Can you work these out from the model? Positions are in its coordinate system, mm. A direction names the side the tool comes from. Coordinates: 2 decimals unless noted, no trailing zeros. Write each loop counter-clockwise with the first axis right and the second up, starting at its lowest first coordinate (ties: lowest second). Pieces come first, ordered by that corner, then holes. Notation, with made-up numbers: (-19.5, 8) -> (9.5, 8) arc R34 cw to (9.5, 40) -> close; hole circle Ø8 at (23.5, 71). An arc over 180 degrees is marked (long way). Use one line per item in the form item = value.
```python
from build123d import *

# Parameters (mm, degrees)
SKETCH1_R           = 1
SKETCH1_R_2         = 0.9
SKETCH1_R_3         = 7.5
BOSS_EXTRUDE1_DEPTH = 1.5
FILLET1_R           = 0.5
CHAMFER1_SIZE       = 0.6


with BuildPart() as part:
    # Sketch1 → Boss-Extrude1 (new body)
    with BuildSketch(Plane(origin=(0, 0, 0), x_dir=(1, 0, 0), z_dir=(0, 1, 0))):
        with BuildLine():
            Line((-10.214212529, -2.433076738), (-12.325317547, -3.651923789))
            ThreePointArc((-12.325317547, -3.651923789), (-13.423393759, -7.75), (-9.325317547, -8.848076211))
            Line((-9.325317547, -8.848076211), (-7.214212529, -7.629229161))
            ThreePointArc((-7.214212529, -7.629229161), (-5.25, -9.09326674), (-3, -10.062305899))
            Line((-3, -10.062305899), (-3, -12.5))
            ThreePointArc((-3, -12.5), (0, -15.5), (3, -12.5))
            Line((3, -12.5), (3, -10.062305899))
            ThreePointArc((3, -10.062305899), (5.25, -9.09326674), (7.214212529, -7.629229161))
            Line((7.214212529, -7.629229161), (9.325317547, -8.848076211))
            ThreePointArc((9.325317547, -8.848076211), (13.423393759, -7.75), (12.325317547, -3.651923789))
            Line((12.325317547, -3.651923789), (10.214212529, -2.433076738))
            ThreePointArc((10.214212529, -2.433076738), (10.410171044, -1.370525018), (10.495898275, -0.293461075))
            Line((10.495898275, -0.293461075), (12.850529964, 0.337460585))
            ThreePointArc((12.850529964, 0.337460585), (14.971850307, 4.011695199), (11.297615693, 6.133015543))
            Line((11.297615693, 6.133015543), (8.942984004, 5.502093883))
            ThreePointArc((8.942984004, 5.502093883), (6.391995005, 8.330210073), (3, 10.062305899))
            Line((3, 10.062305899), (3, 12.5))
            ThreePointArc((3, 12.5), (0, 15.5), (-3, 12.5))
            Line((-3, 12.5), (-3, 10.062305899))
            ThreePointArc((-3, 10.062305899), (-6.391995005, 8.330210073), (-8.942984004, 5.502093883))
            Line((-8.942984004, 5.502093883), (-11.297615693, 6.133015543))
            ThreePointArc((-11.297615693, 6.133015543), (-14.971850307, 4.011695199), (-12.850529964, 0.337460585))
            Line((-12.850529964, 0.337460585), (-10.495898275, -0.293461075))
            ThreePointArc((-10.495898275, -0.293461075), (-10.410171044, -1.370525018), (-10.214212529, -2.433076738))
        make_face()
        with Locations(Location((0, -12.5, 0), (0, 0, 270))):
            Circle(SKETCH1_R, mode=Mode.SUBTRACT)
        with Locations(Location((-10.825317547, -6.25, 0), (0, 0, 270))):
            Circle(SKETCH1_R_2, mode=Mode.SUBTRACT)
        with Locations(Location((10.825317547, -6.25, 0), (0, 0, 270))):
            Circle(SKETCH1_R_2, mode=Mode.SUBTRACT)
        with Locations(Location((0, 0, 0), (0, 0, 270))):
            Circle(SKETCH1_R_3, mode=Mode.SUBTRACT)
        with Locations(Location((0, 12.5, 0), (0, 0, 270))):
            Circle(SKETCH1_R_2, mode=Mode.SUBTRACT)
        with Locations(Location((12.074072829, 3.235238064, 0), (0, 0, 270))):
            Circle(SKETCH1_R, mode=Mode.SUBTRACT)
        with Locations(Location((-12.074072829, 3.235238064, 0), (0, 0, 270))):
            Circle(SKETCH1_R, mode=Mode.SUBTRACT)
    extrude(amount=BOSS_EXTRUDE1_DEPTH)

    # Fillet1
    fillet1_edges = [part.edges().sort_by_distance(p)[0] for p in [
        (-7.214212529, 0.75, 7.629229161),
        (-10.214212529, 0.75, 2.433076738),
        (-10.495898275, 0.75, 0.293461075),
        (-8.942984004, 0.75, -5.502093883),
        (-3, 0.75, -10.062305899),
        (3, 0.75, -10.062305899),
        (8.942984004, 0.75, -5.502093883),
        (10.495898275, 0.75, 0.293461075),
        (10.214212529, 0.75, 2.433076738),
        (7.214212529, 0.75, 7.629229161),
        (3, 0.75, 10.062305899),
        (-3, 0.75, 10.062305899),
    ]]
    fillet(fillet1_edges, radius=FILLET1_R)

    # Chamfer1
    chamfer1_edges = [part.edges().sort_by_distance(p)[0] for p in [
        (10.825317547, 0, 5.35),
        (-10.825317547, 0, 5.35),
        (0, 0, -13.4),
    ]]
    chamfer(chamfer1_edges, length=CHAMFER1_SIZE)


solid = part.part
```
Q1. Suppose I cut it at B-B (z = 6.25). Write out the boundary of the cut face in (x, y).
Return value:
outline = (-13.83, 0) -> (-12.33, 0) -> (-11.73, 0.6) -> (-11.73, 1.5) -> (-13.83, 1.5) -> close; (-9.93, 0.6) -> (-9.33, 0) -> (-4.15, 0) -> (-4.15, 1.5) -> (-9.93, 1.5) -> close; (4.15, 0) -> (9.33, 0) -> (9.93, 0.6) -> (9.93, 1.5) -> (4.15, 1.5) -> close; (11.73, 0.6) -> (12.33, 0) -> (13.83, 0) -> (13.83, 1.5) -> (11.73, 1.5) -> close
Q2. Thinking about a two-plate mould opening in Z: for faces 1 (the cylindrical face through (6.43, 0.74, -8.3)), 2 (the cylindrical face through (-0.6, 0.7, 11.7)), 3 (the cylindrical face through (-13.05, 0.74, -3.45)), 4 (the flat face through (-6, 0, 6)), which applies, released by +Z, released by -Z, zero draft, split by the parting line, or undercut?
Return value:
face_1 = released by -Z
face_2 = undercut
face_3 = undercut
face_4 = zero draft
Q3. Suppose I cut it at C-C (y = 0.9). Give the number of separate pieces and of enclosed holes in the cut face, then the cut area to 3 significant figures.
Return value:
separate_pieces = 1
enclosed_holes = 7
area = 315 mm2
Q4. For faces 5 (the flat face through (11.836, 0.74, -0.066)), 6 (the flat face through (8.416, 0.74, 8.323)), 7 (the flat face through (-10.28, 0.74, -5.86)), 8 (the flat face through (3, 1, 11)), which set-ups out of +Z, -Z, +X, -X, +Y, -Y let a thin tool reach every point of the face, with its end or its side?
Return value:
face_5 = +X, +Y, -Y
face_6 = +Z, +Y, -Y
face_7 = -Z, +Y, -Y
face_8 = +Z, +X, +Y, -Y
Q5. Suppose I cut it at D-D (z = -7). Write out the boundary of the cut face in (x, y), then the cut area to 3 significant figures.
Return value:
outline = (-7.83, 0) -> (-2.69, 0) -> (-2.69, 1.5) -> (-7.83, 1.5) -> close; (2.69, 0) -> (7.83, 0) -> (7.83, 1.5) -> (2.69, 1.5) -> close
area = 15.4 mm2
Q6. If I drill on line 1 (X direction, y = 1.1, z = 8); line 2 (Z direction, x = 11.5, y = 1.1); line 3 (X direction, y = 0.6, z = 12.5), over which ranges is the centre line in solid material (lowest first)? Write a range as from..to.
Return value:
line_1 = -13.26..-7.86, -6.8..6.8, 7.86..13.26
line_2 = -6.18..-4.05, -2.42..0.02, 3.18..5.65, 6.85..9.17
line_3 = -3..-1, 1..3
Q7. Suppose I cut it at A-A (z = 13). Write out the boundary of the cut face in (x, y).
Return value:
outline = (-2.96, 0) -> (-0.87, 0) -> (-0.87, 1.5) -> (-2.96, 1.5) -> close; (0.87, 0) -> (2.96, 0) -> (2.96, 1.5) -> (0.87, 1.5) -> close
